from build123d import *

# Parameters (mm, degrees)
SKETCH1_R           = 10.898656268
SKETCH1_R_2         = 4.749956202
SKETCH1_R_3         = 2.54
BOSS_EXTRUDE1_DEPTH = 5.08


with BuildPart() as part:
    # Sketch1 → Boss-Extrude1 (new body)
    with BuildSketch(Plane.XY):
        Polygon((-73.443857446, -20.706897394), (-73.443857446, -25.786897394), (-80.087904918, -25.786897394), (-80.087904918, -51.975164853), (-73.443857446, -51.975164853), (-73.442970039, -56.866897394), (-22.309257121, -56.866897394), (-22.309257121, -51.786897394), (36.560767605, -51.786897394), (36.560767605, -56.866897394), (87.694480523, -56.866897394), (87.694480523, -51.786897394), (95.535685575, -51.786897394), (95.535685575, -26.395813478), (87.693593116, -25.786897394), (87.693593116, -20.706897394), (36.559880198, -20.706897394), (36.559880198, -25.786897394), (-22.310144528, -25.786897394), (-22.310144528, -20.706897394), align=None)
        with Locations((7.124867835, -38.786897394)):
            Circle(SKETCH1_R, mode=Mode.SUBTRACT)
        with Locations((24.471148926, -38.786897394)):
            Circle(SKETCH1_R_2, mode=Mode.SUBTRACT)
        with Locations((-10.221413257, -38.786897394)):
            Circle(SKETCH1_R_2, mode=Mode.SUBTRACT)
        with Locations((-54.686464291, -33.336890811)):
            Circle(SKETCH1_R_3, mode=Mode.SUBTRACT)
        with Locations((68.93619996, -33.336890811)):
            Circle(SKETCH1_R_3, mode=Mode.SUBTRACT)
        with Locations((68.93619996, -44.236903978)):
            Circle(SKETCH1_R_3, mode=Mode.SUBTRACT)
        with Locations((-54.686464291, -44.236903978)):
            Circle(SKETCH1_R_3, mode=Mode.SUBTRACT)
    extrude(amount=BOSS_EXTRUDE1_DEPTH)


solid = part.part
The model under review builds one solid part; all positions refer to its coordinate system, in mm. A direction names the side the tool comes from. Round coordinates to 2 decimals unless told otherwise and drop trailing zeros. Loops run counter-clockwise (first coordinate to the right, second up) from the corner with the lowest first, then second, coordinate; pieces in that order, holes last. Notation, with made-up numbers: (32, 35) -> (86, 35) arc R34 cw to (86, 66) -> close; hole circle Ø2 at (89, 68). An arc over 180 degrees is marked (long way). Return JSON: item names as keys, results as strings.
(1) Add section A-A on x = 5.5. Write out the cut boundary in (y, z).
Solved:
{"outline": "(-51.79, 0) -> (-49.56, 0) -> (-49.56, 5.08) -> (-51.79, 5.08) -> close; (-28.01, 0) -> (-25.79, 0) -> (-25.79, 5.08) -> (-28.01, 5.08) -> close"}
(2) Add section C-C on z = 0.85. Write out the cut boundary in (x, y).
Solved:
{"outline": "(-80.09, -51.98) -> (-73.44, -51.98) -> (-73.44, -56.87) -> (-22.31, -56.87) -> (-22.31, -51.79) -> (36.56, -51.79) -> (36.56, -56.87) -> (87.69, -56.87) -> (87.69, -51.79) -> (95.54, -51.79) -> (95.54, -26.4) -> (87.69, -25.79) -> (87.69, -20.71) -> (36.56, -20.71) -> (36.56, -25.79) -> (-22.31, -25.79) -> (-22.31, -20.71) -> (-73.44, -20.71) -> (-73.44, -25.79) -> (-80.09, -25.79) -> close; hole circle Ø5.08 at (-54.69, -44.24); hole circle Ø5.08 at (-54.69, -33.34); hole circle Ø9.5 at (-10.22, -38.79); hole circle Ø21.8 at (7.12, -38.79); hole circle Ø9.5 at (24.47, -38.79); hole circle Ø5.08 at (68.94, -44.24); hole circle Ø5.08 at (68.94, -33.34)"}
(3) The part is to be moulded in two halves that separate along X. For faces 1 (the flat face through (87.694, -54, 3)), 2 (the flat face through (-77, -25.787, 3)), 3 (the cylindrical face through (12.15, -48.46, 2.5)), say which applies: released by +X, released by -X, zero draft, split by the parting line, or undercut.
Solved:
{"face 1": "released by +X", "face 2": "zero draft", "face 3": "undercut"}
(4) For line 1 (X direction, y = -39, z = 1.8); line 2 (X direction, y = -35, z = 2.55); line 3 (X direction, y = -36, z = 3.2), list the stretches that pass through material, from the lowest coordinate up.
Solved:
{"line 1": "-80.09 to -14.97, -5.48 to -3.77, 18.02 to 19.73, 29.22 to 95.54", "line 2": "-80.09 to -56.61, -52.77 to -13.09, -7.35 to -3.09, 17.34 to 21.6, 27.34 to 67.02, 70.86 to 95.54", "line 3": "-80.09 to -14.07, -6.37 to -3.41, 17.66 to 20.62, 28.32 to 95.54"}
(5) Add section B-B on x = 70. Write out the cut boundary in (y, z).
Solved:
{"outline": "(-56.87, 0) -> (-46.54, 0) -> (-46.54, 5.08) -> (-56.87, 5.08) -> close; (-41.93, 0) -> (-35.64, 0) -> (-35.64, 5.08) -> (-41.93, 5.08) -> close; (-31.03, 0) -> (-20.71, 0) -> (-20.71, 5.08) -> (-31.03, 5.08) -> close"}
(6) For faces 4 (the flat face through (87.694, -23, 3)), 5 (the flat face through (62, -56.867, 3)), 6 (the flat face through (36.561, -54, 3)), 7 (the flat face through (-22.31, -23, 3)), list the 3-axis set-ups (+Z, -Z, +X, -X, +Y, -Y) from which the entire face can be reached by the end or side of a thin tool; tool diameter is ignored.
Solved:
{"face 4": "+Z, -Z, +X, +Y", "face 5": "+Z, -Z, +X, -X, -Y", "face 6": "+Z, -Z, -Y", "face 7": "+Z, -Z, +Y"}
(7) For pin 1 (17.5 mm diameter, centred on x = 7.12, y = -38.79, fed in from -Z); pin 2 (1.5 mm diameter, centred on x = 19.5, z = 1.5, fed in from -Y); pin 3 (2.5 mm diameter, centred on x = -78, z = 3.5, fed in from +Y); pin 4 (2.5 mm diameter, centred on y = -54.5, z = 3.5, fed in from +X), all flat-tipped, find the tip position at first contact; note any pin that passes through.
Solved:
{"pin 1": "through", "pin 2": "y = -51.79", "pin 3": "y = -25.79", "pin 4": "x = 87.69"}
